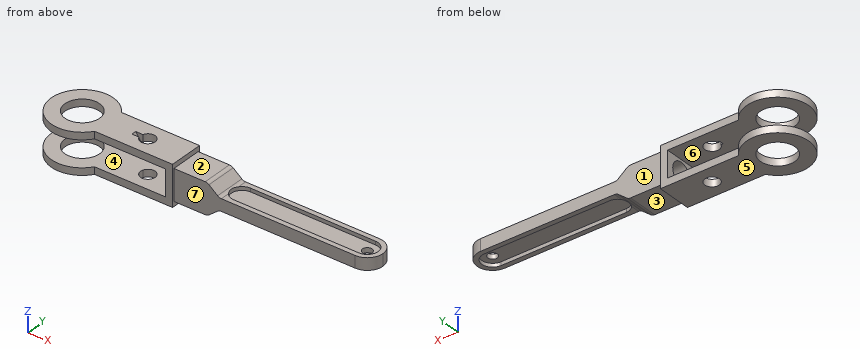
from build123d import *

# Parameters (mm, degrees)
ESBO_O1_R                  = 14.5
RESSALTO_EXTRUS_O1_DEPTH   = 34
CORTE_EXTRUS_O1_DEPTH      = 36
CORTE_EXTRUS_O1_DEPTH_BACK = 56
ESBO_O2_W                  = 115.279866195
ESBO_O2_H                  = 22
RESSALTO_EXTRUS_O2_DEPTH   = 4
RESSALTO_EXTRUS_O3_START   = -6
RESSALTO_EXTRUS_O3_DEPTH   = 6
ESBO_O5_W                  = 26
ESBO_O5_H                  = 26
RESSALTO_EXTRUS_O4_DEPTH   = 28
ESBO_O6_R                  = 9
CORTE_EXTRUS_O2_DEPTH      = 31
ESBO_O7_W                  = 10
ESBO_O7_H                  = 26
RESSALTO_EXTRUS_O5_DEPTH   = 10
RESSALTO_EXTRUS_O7_START   = -26
RESSALTO_EXTRUS_O7_DEPTH   = 26
FILETE1_R                  = 5
ESBO_O9_W                  = 10
ESBO_O9_H                  = 26
RESSALTO_EXTRUS_O8_DEPTH   = 127
FILETE2_R                  = 13
FILETE3_R                  = 5
CORTE_EXTRUS_O3_DEPTH      = 49
CORTE_EXTRUS_O3_DEPTH_BACK = 3
CORTE_EXTRUS_O4_DEPTH      = 52
CORTE_EXTRUS_O4_DEPTH_BACK = 3
CORTE_EXTRUS_O5_DEPTH      = 27
CORTE_EXTRUS_O5_DEPTH_BACK = 22
ESBO_O12_R                 = 4


with BuildPart() as part:
    # Esboço1 → Ressalto-extrusão1 (new body)
    with BuildSketch(Plane.XY):
        with BuildLine():
            Line((21.581241855, 14.5), (87, 14.5))
            Line((87, 14.5), (87, -14.5))
            Line((87, -14.5), (21.581241855, -14.5))
            ThreePointArc((21.581241855, -14.5), (-26, 0), (21.581241855, 14.5))
        make_face()
        Circle(ESBO_O1_R, mode=Mode.SUBTRACT)
        with BuildLine():
            ThreePointArc((49.210731912, -2), (61.125, 0), (49.210731912, 2))
            Line((49.210731912, 2), (43.210731912, 2))
            Line((43.210731912, 2), (43.210731912, -2))
            Line((43.210731912, -2), (49.210731912, -2))
        make_face(mode=Mode.SUBTRACT)
    extrude(amount=RESSALTO_EXTRUS_O1_DEPTH)

    # Esboço2 → Corte-extrusão1 (cut, two sides: drawn at the far end of the back side and taken through both)
    with BuildSketch(Plane(origin=(0, 14.5, 0), x_dir=(1, 0, 0), z_dir=(0, 1, 0)).offset(-CORTE_EXTRUS_O1_DEPTH_BACK)):
        with Locations((23.360066902, -17)):
            Rectangle(ESBO_O2_W, ESBO_O2_H)
    extrude(amount=CORTE_EXTRUS_O1_DEPTH + CORTE_EXTRUS_O1_DEPTH_BACK, mode=Mode.SUBTRACT)

    # Esboço3 → Ressalto-extrusão2 (add)
    with BuildSketch(Plane(origin=(0, -2, 0), x_dir=(1, 0, 0), z_dir=(0, 1, 0))):
        Polygon((43.210731912, -28), (47.210731912, -28), (43.210731912, -34), align=None)
    extrude(amount=RESSALTO_EXTRUS_O2_DEPTH)

    # Esboço4 → Ressalto-extrusão3 (add)
    with BuildSketch(Plane.XY.offset(6).offset(RESSALTO_EXTRUS_O3_START)):
        with BuildLine():
            ThreePointArc((49.210731912, 2), (48.875, 0), (49.210731912, -2))
            Line((49.210731912, -2), (43.210731912, -2))
            Line((43.210731912, -2), (43.210731912, 2))
            Line((43.210731912, 2), (49.210731912, 2))
        make_face()
    extrude(amount=RESSALTO_EXTRUS_O3_DEPTH)

    # Esboço5 → Ressalto-extrusão4 (add)
    with BuildSketch(Plane(origin=(87, 0, 0), x_dir=(0, 0, -1), z_dir=(1, 0, 0))):
        with Locations((-17, 0)):
            Rectangle(ESBO_O5_W, ESBO_O5_H)
    extrude(amount=RESSALTO_EXTRUS_O4_DEPTH)

    # Esboço6 → Corte-extrusão2 (cut)
    with BuildSketch(Plane.ZY.offset(-81)):
        with Locations((17, 0)):
            Circle(ESBO_O6_R)
    extrude(amount=-CORTE_EXTRUS_O2_DEPTH, mode=Mode.SUBTRACT)

    # Esboço7 → Ressalto-extrusão5 (add)
    with BuildSketch(Plane(origin=(115, 0, 0), x_dir=(0, 0, -1), z_dir=(1, 0, 0))):
        with Locations((-17, 0)):
            Rectangle(ESBO_O7_W, ESBO_O7_H)
    extrude(amount=RESSALTO_EXTRUS_O5_DEPTH)

    # Esboço8 → Ressalto-extrusão7 (add)
    with BuildSketch(Plane(origin=(0, 13, 0), x_dir=(1, 0, 0), z_dir=(0, 1, 0)).offset(RESSALTO_EXTRUS_O7_START)):
        Polygon((125, -12), (115, -4), (115, -12), align=None)
        Polygon((125, -22), (115, -22), (115, -30), align=None)
    extrude(amount=RESSALTO_EXTRUS_O7_DEPTH)

    # Filete1
    filete1_edges = [part.edges().sort_by_distance(p)[0] for p in [
        (115, 0, 30),
        (115, 0, 4),
    ]]
    fillet(filete1_edges, radius=FILETE1_R)

    # Esboço9 → Ressalto-extrusão8 (add)
    with BuildSketch(Plane(origin=(125, 0, 0), x_dir=(0, 0, -1), z_dir=(1, 0, 0))):
        with Locations((-17, 0)):
            Rectangle(ESBO_O9_W, ESBO_O9_H)
    extrude(amount=RESSALTO_EXTRUS_O8_DEPTH)

    # Filete2
    filete2_edges = [part.edges().sort_by_distance(p)[0] for p in [
        (252, -13, 17),
        (252, 13, 17),
    ]]
    fillet(filete2_edges, radius=FILETE2_R - 0.0001)  # a hair under: the kernel refuses the full size

    # Filete3
    filete3_edges = [part.edges().sort_by_distance(p)[0] for p in [
        (125, 0, 22),
        (125, 0, 12),
    ]]
    fillet(filete3_edges, radius=FILETE3_R)

    # Esboço10 → Corte-extrusão3 (cut, two sides: drawn at the far end of the back side and taken through both)
    with BuildSketch(Plane.XY.offset(22).offset(-CORTE_EXTRUS_O3_DEPTH_BACK)):
        with BuildLine():
            Line((134, 9), (239, 9))
            ThreePointArc((239, 9), (248, 0), (239, -9))
            Line((239, -9), (134, -9))
            ThreePointArc((134, -9), (125, 0), (134, 9))
        make_face()
    extrude(amount=CORTE_EXTRUS_O3_DEPTH + CORTE_EXTRUS_O3_DEPTH_BACK, mode=Mode.SUBTRACT)

    # Esboço11 → Corte-extrusão4 (cut, two sides: drawn at the far end of the back side and taken through both)
    with BuildSketch(Plane(origin=(0, 0, 12), x_dir=(-1, 0, 0), z_dir=(0, 0, -1)).offset(-CORTE_EXTRUS_O4_DEPTH_BACK)):
        with BuildLine():
            Line((-239, 9), (-134, 9))
            ThreePointArc((-134, 9), (-125, 0), (-134, -9))
            Line((-134, -9), (-239, -9))
            ThreePointArc((-239, -9), (-248, 0), (-239, 9))
        make_face()
    extrude(amount=CORTE_EXTRUS_O4_DEPTH + CORTE_EXTRUS_O4_DEPTH_BACK, mode=Mode.SUBTRACT)

    # Esboço12 → Corte-extrusão5 (cut, two sides: drawn at the far end of the back side and taken through both)
    with BuildSketch(Plane(origin=(0, 0, 15), x_dir=(-1, 0, 0), z_dir=(0, 0, -1)).offset(-CORTE_EXTRUS_O5_DEPTH_BACK)):
        with Locations(Location((-239, 0, 0), (0, 0, 180))):
            Circle(ESBO_O12_R)
    extrude(amount=CORTE_EXTRUS_O5_DEPTH + CORTE_EXTRUS_O5_DEPTH_BACK, mode=Mode.SUBTRACT)


solid = part.part
Check sheet for the modelled part. Datum: model origin and axes. Units: mm. Face numbers are marked on the shaded views. A direction names the side the tool comes from. Give positions to 0.01 mm unless a question says otherwise; leave off trailing zeros. Write each loop counter-clockwise with the first axis right and the second up, starting at its lowest first coordinate (ties: lowest second). Pieces come first, ordered by that corner, then holes. Notation, with made-up numbers: M -0.75,27.5 L 43.25,27.5 A24 ccw 43.25,62.5 Z; hole C 28,62.25 d2. An arc over 180 degrees is marked long. Use one line per item in the form item = value.
(1) Section check A-A on x = 0. Record the boundary of the cut face in (y, z), plus the area to 3 significant figures.
Answer block:
outline = M -26,0 L -14.5,0 L -14.5,6 L -26,6 Z; M -26,28 L -14.5,28 L -14.5,34 L -26,34 Z; M 14.5,0 L 26,0 L 26,6 L 14.5,6 Z; M 14.5,28 L 26,28 L 26,34 L 14.5,34 Z
area = 276 mm2
(2) Section check B-B on x = 180.5. Record the boundary of the cut face in (y, z).
Answer block:
outline = M -13,12 L -9,12 L -9,15 L 9,15 L 9,12 L 13,12 L 13,22 L 9,22 L 9,19 L -9,19 L -9,22 L -13,22 Z
(3) Tool access check on the marked faces 1, 2 and 3. Record the directions out of +Z, -Z, +X, -X, +Y, -Y that give a thin tool (end or side, any length) a straight path to the whole face; none if there is none.
Answer block:
face_1 = +Z, -Z, +X, +Y
face_2 = +Z, +X, +Y, -Y
face_3 = -Z, +X, +Y, -Y
(4) Section check D-D on x = 55. Record the boundary of the cut face in (y, z) (3 decimals).
Answer block:
outline = M -14.5,0 L -6.125,0 L -6.125,6 L -14.5,6 Z; M -14.5,28 L -6.125,28 L -6.125,34 L -14.5,34 Z; M 6.125,0 L 14.5,0 L 14.5,6 L 6.125,6 Z; M 6.125,28 L 14.5,28 L 14.5,34 L 6.125,34 Z
(5) Draft check along Z on the marked faces 4, 5, 6 and 7. Enter one of: pulls with the +Z half, pulls with the -Z half, needs draft (parallel to the pull), parting line crosses it, or undercut.
Answer block:
face_4 = undercut
face_5 = pulls with the -Z half
face_6 = undercut
face_7 = needs draft
(6) Material ranges on line 1 along Y through (x, z) = (239, 15.9); line 2 along Y through (x, z) = (55, 32.2) (3 decimals); line 3 along Z through (x, y) = (66, 6), recorded low to high.
Answer block:
line_1 = -13 to -4, 4 to 13
line_2 = -14.5 to -6.125, 6.125 to 14.5
line_3 = 0 to 6, 28 to 34
(7) Section check C-C on x = 96.5. Record the boundary of the cut face in (y, z), plus the area to 3 significant figures.
Answer block:
outline = M -13,4 L 13,4 L 13,30 L -13,30 Z; hole C 0,17 d18
area = 422 mm2
(8) Depth check by flat-ended pin: P1, Ø5, axis at y = 6, z = 5.5, coming from the -X side; P2, Ø1.8, axis at x = 47.5, z = 30.5, coming from the -Y side; P3, Ø16, axis at x = 55, y = 0, coming from the +Z side; P4, Ø9, axis at x = 217, y = -2.5, coming from the -Z side. Enter the tip coordinate at first touch or a pass-through.
Answer block:
P1 = -25.76
P2 = -14.5
P3 = 34
P4 = 15
